Geometry: final body of the model. Coordinates: model frame, mm. Face numbers are marked on the shaded views. A direction names the side the tool comes from. Round coordinates to 2 decimals unless told otherwise and drop trailing zeros. Write each loop counter-clockwise with the first axis right and the second up, starting at its lowest first coordinate (ties: lowest second). Pieces come first, ordered by that corner, then holes.
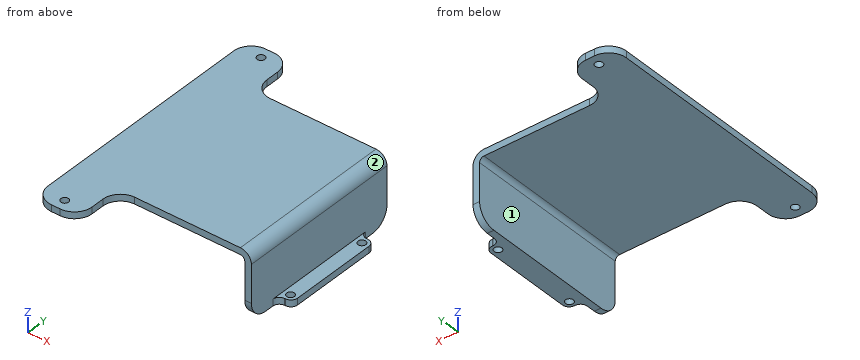
from build123d import *

# Parameters (mm, degrees)
ESQUISSE1_R             = 1.75
BOSS_EXTRU_1_DEPTH      = 3
ESQUISSE1_3_W           = 6.4
ESQUISSE1_3_H           = 46
ESQUISSE1_3_R           = 1.75
BOSS_EXTRU_2_DEPTH      = 27
ESQUISSE1_4_W           = 6.4
ESQUISSE1_4_H           = 46
ESQUISSE1_4_R           = 1.75
ENL_V_MAT_EXTRU_1_DEPTH = 24
CONG_1_R                = 8
CONG_2_R                = 3
CONG_3_R                = 2
CONG_4_R                = 5


with BuildPart() as part:
    # Esquisse1 → Boss.-Extru.1 (new body)
    with BuildSketch(Plane.XY):
        Polygon((30.5, 38), (-30.5, 38), (-30.5, 60), (-50.5, 60), (-50.5, -60), (-30.5, -60), (-30.5, -38), (30.5, -38), align=None)
        with Locations((-40.5, 55)):
            Circle(ESQUISSE1_R, mode=Mode.SUBTRACT)
        with Locations((-40.5, -55)):
            Circle(ESQUISSE1_R, mode=Mode.SUBTRACT)
    extrude(amount=BOSS_EXTRU_1_DEPTH)

    # Esquisse1_3 → Boss.-Extru.2 (add)
    with BuildSketch(Plane.XY):
        Polygon((30.5, -23), (30.5, 23), (30.5, 38), (27.5, 38), (27.5, -38), (30.5, -38), align=None)
        with Locations((33.7, 0)):
            Rectangle(ESQUISSE1_3_W, ESQUISSE1_3_H)
        with Locations((33.7, -20)):
            Circle(ESQUISSE1_3_R, mode=Mode.SUBTRACT)
        with Locations((33.7, 20)):
            Circle(ESQUISSE1_3_R, mode=Mode.SUBTRACT)
    extrude(amount=-BOSS_EXTRU_2_DEPTH)

    # Esquisse1_4 → Enl_v. mat.-Extru.1 (cut)
    with BuildSketch(Plane.XY):
        with Locations((33.7, 0)):
            Rectangle(ESQUISSE1_4_W, ESQUISSE1_4_H)
        with Locations((33.7, -20)):
            Circle(ESQUISSE1_4_R, mode=Mode.SUBTRACT)
        with Locations((33.7, 20)):
            Circle(ESQUISSE1_4_R, mode=Mode.SUBTRACT)
    extrude(amount=-ENL_V_MAT_EXTRU_1_DEPTH, mode=Mode.SUBTRACT)

    # Cong_1
    cong_1_edges = [part.edges().sort_by_distance(p)[0] for p in [
        (-50.5, -60, 1.5),
        (-50.5, 60, 1.5),
        (-30.5, 60, 1.5),
        (-30.5, 38, 1.5),
        (-30.5, -38, 1.5),
        (-30.5, -60, 1.5),
        (29, -38, -27),
        (29, 38, -27),
    ]]
    fillet(cong_1_edges, radius=CONG_1_R)

    # Cong_2
    cong_2_edges = [part.edges().sort_by_distance(p)[0] for p in [
        (30.5, 23, -25.5),
        (36.9, 23, -25.5),
        (36.9, -23, -25.5),
        (30.5, -23, -25.5),
    ]]
    fillet(cong_2_edges, radius=CONG_2_R)

    # Cong_3
    cong_3_edges = [part.edges().sort_by_distance(p)[0] for p in [
        (27.5, 0, 0),
    ]]
    fillet(cong_3_edges, radius=CONG_3_R)

    # Cong_4
    cong_4_edges = [part.edges().sort_by_distance(p)[0] for p in [
        (30.5, 0, 3),
    ]]
    fillet(cong_4_edges, radius=CONG_4_R)


solid = part.part
1) Section D-D on z = -8. Output: boundary loops of the cut face in (x, y).
2) First-contact query: P1, Ø3, axis at y = -1.5, z = -8, coming from the +X side; P2, Ø1.5, axis at y = 49, z = 2, coming from the +X side; P3, Ø3, axis at x = -40.5, y = 55, coming from the +Z side; P4, Ø1.5, axis at y = 26, z = -23, coming from the -X side. Flat tips, straight axial feed; report the tip coordinate or a pass-through.
3) Reachability of the marked faces 1 and 2 from +Z, -Z, +X, -X, +Y, -Y: full face, straight path, thin tool, end or side. Return the list, or none.
4) Section B-B on y = -28. Output: boundary loops of the cut face in (x, z).
5) Section C-C on y = 55. Output: boundary loops of the cut face in (x, z).
6) Line query: probe 1 along Y at (x, z) = (33.7, -25.5); probe 2 along Y at (x, z) = (-40.5, 1.45); probe 3 along X at (y, z) = (-20, -23.75). Output: solid intervals per line, ascending.
7) Section A-A on x = -40.5. Output: boundary loops of the cut face in (y, z), plus the area to 3 significant figures.
Filled in:
1. outline: (27.5, -38) - (30.5, -38) - (30.5, 38) - (27.5, 38) - close
2. P1: stops at x = 30.5
2. P2: stops at x = -30.5
2. P3: passes through
2. P4: stops at x = 27.5
3. face 1: -Z, -X, +Y, -Y
3. face 2: +Z, +X, +Y, -Y
4. outline: (-50.5, 0) - (25.5, 0) arc R2 cw to (27.5, -2) - (27.5, -27) - (30.5, -27) - (30.5, -2) arc R5 ccw to (25.5, 3) - (-50.5, 3) - close
5. outline: (-49.92, 0) - (-42.25, 0) - (-42.25, 3) - (-49.92, 3) - close; (-38.75, 0) - (-31.08, 0) - (-31.08, 3) - (-38.75, 3) - close
6. probe 1: y = -23 to -21.75, -18.25 to 18.25, 21.75 to 23
6. probe 2: y = -60 to -56.75, -53.25 to 53.25, 56.75 to 60
6. probe 3: x = 27.5 to 30.5
7. outline: (-60, 0) - (-56.75, 0) - (-56.75, 3) - (-60, 3) - close; (-53.25, 0) - (53.25, 0) - (53.25, 3) - (-53.25, 3) - close; (56.75, 0) - (60, 0) - (60, 3) - (56.75, 3) - close
7. area: 339 mm2
